Answer from the drawing. Dimensions are ordinates in mm from the lowest x, y and z of the part. Coordinates: 2 decimals unless noted, no trailing zeros. Order: outer loops, then holes, each group sorted by start corner. A loop starts at its lowest first (then second) coordinate and runs counter-clockwise, first axis right, second up. Notation, with made-up numbers: M -39,-3.75 L 5,-3.75 A21 ccw 5,26.25 Z; hole C 1.25,4.5 d6. An arc over 180 degrees is marked long. Use a Markdown table: item, result.
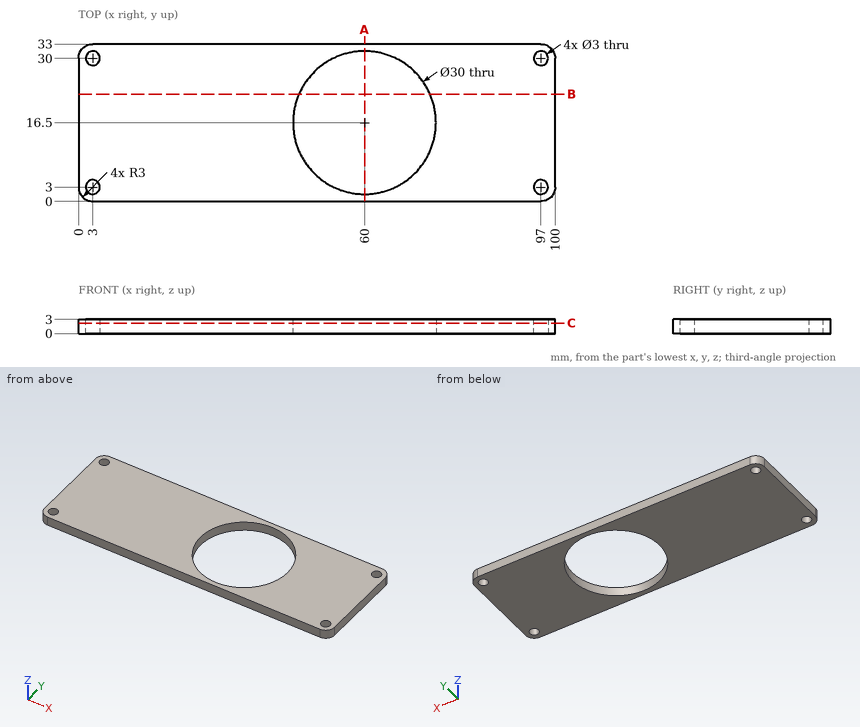
(1) Given P1, Ø3.5, axis at x = 3, y = 30, coming from the +Z side, flat-ended and moving along its own axis, determine where the tip first touches the part or whether it passes through.
Conclusion:
| item | result |
|---|---|
| P1 | z = 3 |
(2) A cutting plane is placed at B-B (y = 22.5). Determine the outline of the cut face in (x, z), then the cut area to 3 significant figures.
Conclusion:
| item | result |
|---|---|
| outline | M 0,0 L 46.25,0 L 46.25,3 L 0,3 Z; M 73.75,0 L 100,0 L 100,3 L 73.75,3 Z |
| area | 218 mm2 |
(3) A cutting plane is placed at C-C (z = 2.2). Determine the outline of the cut face in (x, y), then the cut area to 3 significant figures.
Conclusion:
| item | result |
|---|---|
| outline | M 0,3 A3 ccw 3,0 L 97,0 A3 ccw 100,3 L 100,30 A3 ccw 97,33 L 3,33 A3 ccw 0,30 Z; hole C 3,3 d3; hole C 3,30 d3; hole C 60,16.5 d30; hole C 97,3 d3; hole C 97,30 d3 |
| area | 2,560 mm2 |
(4) A cutting plane is placed at A-A (x = 60). Determine the outline of the cut face in (y, z).
Conclusion:
| item | result |
|---|---|
| outline | M 0,0 L 1.5,0 L 1.5,3 L 0,3 Z; M 31.5,0 L 33,0 L 33,3 L 31.5,3 Z |
(5) Straight lines are drawn through the part: L1, parallel to Y at x = 97, z = 1.6; L2, parallel to Y at x = 60, z = 2.3; L3, parallel to Y at x = 57.5, z = 1.7. For each, find the intervals that lie inside material, in ascending order.
Conclusion:
| item | result |
|---|---|
| L1 | 0 to 1.5, 4.5 to 28.5, 31.5 to 33 |
| L2 | 0 to 1.5, 31.5 to 33 |
| L3 | 0 to 1.71, 31.29 to 33 |
